Model file for the job. Use its own axes, mm. Face numbers are marked on the shaded views. A direction names the side the tool comes from. Coordinates: 2 decimals unless noted, no trailing zeros. Loops run counter-clockwise (first coordinate to the right, second up) from the corner with the lowest first, then second, coordinate; pieces in that order, holes last. Notation, with made-up numbers: (-21.5, 39) -> (-0.5, 39) arc R23 ccw to (-0.5, 55) -> close; hole circle Ø9 at (-14.5, -40). An arc over 180 degrees is marked (long way). Use one line per item in the form item = value.
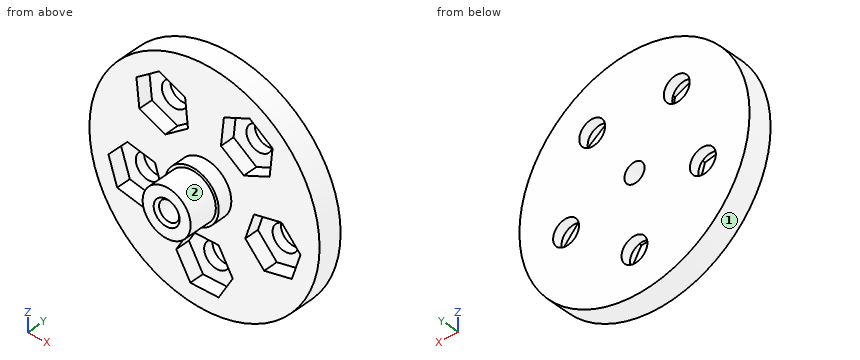
Autodesk Inventor part; units mm, degrees
ref_plane "YZ Plane" through (0, 0, 0) normal (1, 0, 0) x (0, 1, 0)
ref_plane "XZ Plane" through (0, 0, 0) normal (0, 1, 0) x (-1, 0, 0)
ref_plane "XY Plane" through (0, 0, 0) normal (0, 0, 1) x (1, 0, 0)
sketch "Sketch1" plane through (0, 0, 0) normal (0, 0, 1) x (1, 0, 0)
  line L0 (0, 7) -> (0, 0) construction
  line L1 (0, 0) -> (1.05, 0) construction
  line L2 (1.05, 0) -> (1.05, 7)
  line L3 (1.05, 7) -> (0, 7) construction
  line L4 (1.05, 7) -> (12, 7)
  line L5 (2.8, 3) -> (2.5, 3)
  line L6 (2.5, 3) -> (2.5, 0)
  line L7 (2.5, 0) -> (1.05, 0)
  line L8 (12, 7) -> (12, 4.5)
  line L9 (12, 4.5) -> (2.8, 4.5)
  line L10 (2.8, 4.5) -> (2.8, 3)
  dimension "d0" = 2.5
  dimension "d1" = 1.05
  dimension "d3" = 0.3
  dimension "d4" = 3
  dimension "d9" = 1.5
  dimension "d10" = 12
  dimension "d11" = 2.5
revolve "Revolution1" add sketch "Sketch1" angle 360 about axis through (0, 7, 0) along (0, -1, 0)
sketch "Sketch2" plane through (0, 7, 0) normal (0, 1, 0) x (1, 0, 0)
  line L0 (0, 0) -> (0, 7.5) construction
  circle A0 centre (0, 7.5) radius 1.35
  line L1 (0, 0) -> (-7.1329, 2.3176) construction
  circle A1 centre (-7.1329, 2.3176) radius 1.35
  line L2 (0, 0) -> (-4.4084, -6.0676) construction
  circle A2 centre (-4.4084, -6.0676) radius 1.35
  line L3 (0, 0) -> (4.4084, -6.0676) construction
  circle A3 centre (4.4084, -6.0676) radius 1.35
  line L4 (0, 0) -> (7.1329, 2.3176) construction
  circle A4 centre (7.1329, 2.3176) radius 1.35
  dimension "d12" = 7.5
  dimension "d13" = 2.7
  dimension "d16" = 360
extrude "Extrusion1" cut sketch "Sketch2" against normal blind 10
sketch "Sketch3" plane through (0, 4.5, 0) normal (0, -1, 0) x (1, 0, 0)
  circle A0 centre (0, -7.5) radius 1.35 construction
  line L0 (-2.9445, -7.5) -> (-1.4722, -4.95)
  line L1 (-1.4722, -4.95) -> (1.4722, -4.95)
  line L2 (1.4722, -4.95) -> (2.9445, -7.5)
  line L3 (2.9445, -7.5) -> (1.4722, -10.05)
  line L4 (1.4722, -10.05) -> (-1.4722, -10.05)
  line L5 (-1.4722, -10.05) -> (-2.9445, -7.5)
  line L6 (6.223, -5.118) -> (4.2528, -2.9298)
  line L7 (4.2528, -2.9298) -> (5.1627, -0.1294)
  line L8 (5.1627, -0.1294) -> (8.0428, 0.4827)
  line L9 (8.0428, 0.4827) -> (10.0131, -1.7054)
  line L10 (10.0131, -1.7054) -> (9.1032, -4.5058)
  line L11 (9.1032, -4.5058) -> (6.223, -5.118)
  line L12 (6.7905, 4.3369) -> (4.1006, 3.1393)
  line L13 (4.1006, 3.1393) -> (1.7185, 4.87)
  line L14 (1.7185, 4.87) -> (2.0262, 7.7984)
  line L15 (2.0262, 7.7984) -> (4.7162, 8.996)
  line L16 (4.7162, 8.996) -> (7.0983, 7.2653)
  line L17 (7.0983, 7.2653) -> (6.7905, 4.3369)
  line L18 (-2.0262, 7.7984) -> (-1.7185, 4.87)
  line L19 (-1.7185, 4.87) -> (-4.1006, 3.1393)
  line L20 (-4.1006, 3.1393) -> (-6.7905, 4.3369)
  line L21 (-6.7905, 4.3369) -> (-7.0983, 7.2653)
  line L22 (-7.0983, 7.2653) -> (-4.7162, 8.996)
  line L23 (-4.7162, 8.996) -> (-2.0262, 7.7984)
  line L24 (-8.0428, 0.4827) -> (-5.1627, -0.1294)
  line L25 (-5.1627, -0.1294) -> (-4.2528, -2.9298)
  line L26 (-4.2528, -2.9298) -> (-6.223, -5.118)
  line L27 (-6.223, -5.118) -> (-9.1032, -4.5058)
  line L28 (-9.1032, -4.5058) -> (-10.0131, -1.7054)
  line L29 (-10.0131, -1.7054) -> (-8.0428, 0.4827)
  point P0 (0, 0)
  point P1 (0, -7.5)
  point P2 (7.1329, -2.3176)
  point P3 (7.1329, -2.3176)
  point P4 (4.4084, 6.0676)
  point P5 (4.4084, 6.0676)
  point P6 (-4.4084, 6.0676)
  point P7 (-4.4084, 6.0676)
  point P8 (-7.1329, -2.3176)
  point P9 (-7.1329, -2.3176)
  dimension "d20" = 5.1
  dimension "d23" = 360
extrude "Extrusion2" cut sketch "Sketch3" against normal blind 1.5
chamfer "Chamfer2" distance 0.3 angle 45 1 edges at (-1.05, 0, 0)
properties part number "Flywheel"
Q1. Which spindle directions (+Z, -Z, +X, -X, +Y, -Y) get a long thin tool onto all of the face, cutting with end or side? Do the marked faces 1 and 2. Say none if no direction does.
Result:
face_1 = +Y, -Y
face_2 = -Y
Q2. Band-saw the part on C-C, the plane y = 3.5. Write the cut outline in (x, z).
Result:
outline = circle Ø5.6 at (0, 0); hole circle Ø2.1 at (0, 0)
Q3. Wall check: line 1 along Z through (x, y) = (0, 5.25); line 2 along Z through (x, y) = (0, 6.2); line 3 along Y through (x, z) = (-0.5, -3.25). Give the ranges that are in metal, low to high.
Result:
line_1 = -12 to -10.05, -4.95 to -1.05, 1.05 to 12
line_2 = -12 to -8.85, -6.15 to -1.05, 1.05 to 12
line_3 = 4.5 to 7
Q4. Band-saw the part on A-A, the plane x = 0. Write the cut outline in (y, z).
Result:
outline = (0, -2.5) -> (3, -2.5) -> (3, -2.8) -> (4.5, -2.8) -> (4.5, -4.95) -> (6, -4.95) -> (6, -6.15) -> (7, -6.15) -> (7, -1.05) -> (0.3, -1.05) -> (0, -1.35) -> close; (0, 1.35) -> (0.3, 1.05) -> (7, 1.05) -> (7, 12) -> (4.5, 12) -> (4.5, 2.8) -> (3, 2.8) -> (3, 2.5) -> (0, 2.5) -> close; (4.5, -12) -> (7, -12) -> (7, -8.85) -> (6, -8.85) -> (6, -10.05) -> (4.5, -10.05) -> close
Q5. Band-saw the part on B-B, the plane x = -7.5. Write the cut outline in (y, z).
Result:
outline = (4.5, -9.37) -> (7, -9.37) -> (7, -3.62) -> (6, -3.62) -> (6, -4.85) -> (4.5, -4.85) -> close; (4.5, 0.37) -> (6, 0.37) -> (6, -1.02) -> (7, -1.02) -> (7, 9.37) -> (4.5, 9.37) -> close
Q6. Pin check, flat tips, straight feed: pin 1 Ø1.6 at (x, z) = (-5, 6.5) entering from -Y; pin 2 Ø4 at (x, y) = (3.5, 5) entering from +Z; pin 3 Ø1.5 at (x, y) = (6, 4.5) entering from +Z; pin 4 Ø1.3 at (x, z) = (0, 0) entering from +Y. Stop position of each tip, or through.
Result:
pin_1 = 6
pin_2 = 11.91
pin_3 = 10.79
pin_4 = through
Q7. Band-saw the part on D-D, the plane y = 2. Write the cut outline in (x, z).
Result:
outline = circle Ø5 at (0, 0); hole circle Ø2.1 at (0, 0)
